```python
from build123d import *

# Parameters (mm, degrees)
SKETCH1_W           = 83
SKETCH1_H           = 100
BOSS_EXTRUDE1_DEPTH = 0.5
M2_HOLE1_A_D        = 2.4


with BuildPart() as part:
    # Sketch1 → Boss-Extrude1 (new, symmetric)
    with BuildSketch(Plane.XY):
        Rectangle(SKETCH1_W, SKETCH1_H)
    extrude(amount=BOSS_EXTRUDE1_DEPTH, both=True)

    # M2 Hole1 - A (through all)
    with Locations(Plane.XY.offset(0.5)):
        with Locations((-35.5, 47.5), (35.5, 47.5), (-35.5, -47.5), (35.5, -47.5)):
            Hole(M2_HOLE1_A_D / 2)


solid = part.part
```
The listing builds one solid part. Answer for the finished solid, in the listing's coordinates (mm). Round coordinates to 2 decimals unless told otherwise and drop trailing zeros. Order: outer loops, then holes, each group sorted by start corner. A loop starts at its lowest first (then second) coordinate and runs counter-clockwise, first axis right, second up. Notation, with made-up numbers: (29.5, 69.25) -> (65.5, 69.25) arc R17 ccw to (65.5, 85.25) -> close; hole circle Ø2 at (74, -28). An arc over 180 degrees is marked (long way). Answer as CSV lines item,"result".
Q1. Given pin 1 (3 mm diameter, centred on x = 35.5, y = -47.5, fed in from +Z), flat-ended and moving along its own axis, determine where the tip first touches the part or whether it passes through.
Computed values:
pin 1,"stops at z = 0.5"
Q2. Consider line 1 (Y direction, x = -35.5, z = 0.1); line 2 (Y direction, x = 36.5, z = 0.1). Determine where each line is inside the solid, lowest interval first. Write a range as from..to.
Computed values:
line 1,"y = -50..-48.7, -46.3..46.3, 48.7..50"
line 2,"y = -50..-48.16, -46.84..46.84, 48.16..50"
Q3. A cutting plane is placed at B-B on y = -47.5. Determine the outline of the cut face in (x, z), plus the area to 3 significant figures.
Computed values:
outline,"(-41.5, -0.5) -> (-36.7, -0.5) -> (-36.7, 0.5) -> (-41.5, 0.5) -> close; (-34.3, -0.5) -> (34.3, -0.5) -> (34.3, 0.5) -> (-34.3, 0.5) -> close; (36.7, -0.5) -> (41.5, -0.5) -> (41.5, 0.5) -> (36.7, 0.5) -> close"
area,"78.2 mm^2"
Q4. For a pull along Y with two mould halves and no side action, classify faces 1 (the flat face through (-1, 1, -0.5)), 2 (the cylindrical face through (34.85, -46.49, -0.01)) as +Y half, -Y half, draft (parallel to the pull), parting line (faces both ways), or undercut.
Computed values:
face 1,"draft"
face 2,"undercut"
Q5. A cutting plane is placed at A-A on x = 35.5. Determine the outline of the cut face in (y, z).
Computed values:
outline,"(-50, -0.5) -> (-48.7, -0.5) -> (-48.7, 0.5) -> (-50, 0.5) -> close; (-46.3, -0.5) -> (46.3, -0.5) -> (46.3, 0.5) -> (-46.3, 0.5) -> close; (48.7, -0.5) -> (50, -0.5) -> (50, 0.5) -> (48.7, 0.5) -> close"
